Geometry: see drawing. Coordinates: mm, zero at the bounding-box minimum. A direction names the side the tool comes from. Give positions to 0.01 mm unless a question says otherwise; leave off trailing zeros. Loops run counter-clockwise (first coordinate to the right, second up) from the corner with the lowest first, then second, coordinate; pieces in that order, holes last. Notation, with made-up numbers: (89.5, 14.5) -> (94.5, 14.5) arc R33 ccw to (94.5, 44.5) -> close; hole circle Ø5 at (38.5, -7.5). An arc over 180 degrees is marked (long way). Return JSON: item names as keys, results as strings. Group by question number.
(1) Draft query along X for the marked faces 3, 4 and 5. Return one class per face: released by +X, released by -X, zero draft, split by the parting line, or undercut.
(2) Ray query, line 1 (X direction, y = 1.75, z = 10.5); line 2 (X direction, y = 5.75, z = 5.5); line 3 (X direction, y = 3.5, z = 7.75). Return the intervals inside material, ascending. Write a range as from..to.
(3) Cut plane C-C on y = 2.25. Return loops of the section in (x, z), then the cut area to 3 significant figures.
(4) Cut plane B-B on z = 3.5. Return loops of the section in (x, y).
(5) Pin query (flat end, axial travel): pin 1 (2 mm diameter, centred on y = 3, z = 3, fed in from -X); pin 2 (0.5 mm diameter, centred on y = 2, z = 6, fed in from -X); pin 3 (0.9 mm diameter, centred on y = 5, z = 0.5, fed in from -X); pin 4 (3.5 mm diameter, centred on x = 60, y = 2.5, fed in from +Z). Return the tip coordinate at first contact, or that it passes through.
(6) Cut plane D-D on x = 36. Return loops of the section in (y, z).
(7) Cut plane A-A on x = 3.5. Return loops of the section in (y, z).
(8) Access query for the marked faces 1 and 2. Directions: +Z, -Z, +X, -X, +Y, -Y. A direction counts if a zero-diameter tool reaches every point of the face in a straight line with its end or side. Return the directions, or none.
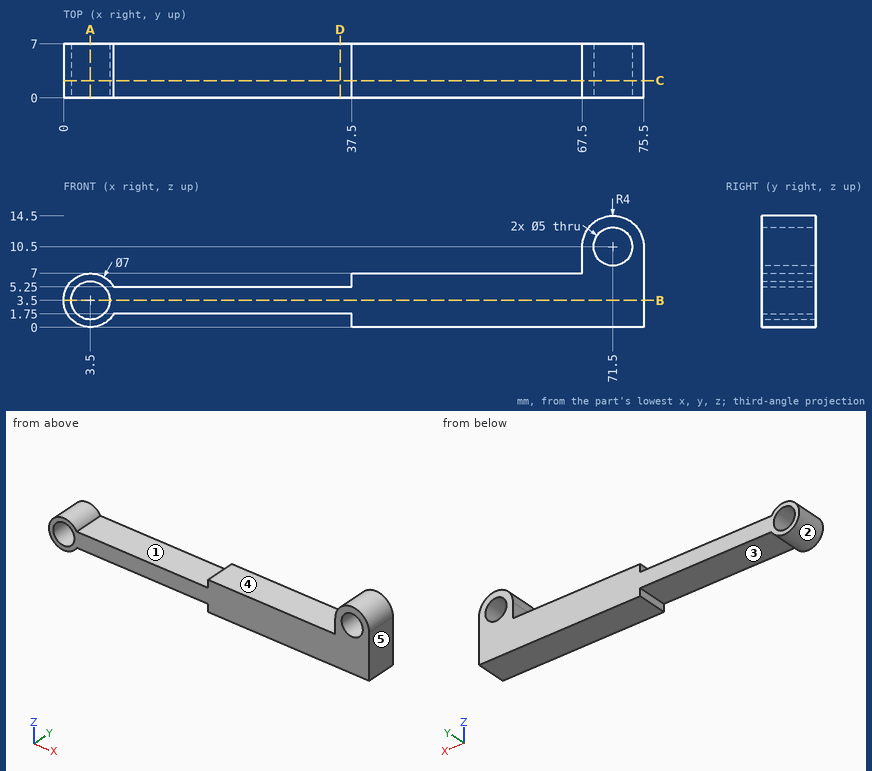
Answers:
{
 "1": {"face 3": "undercut", "face 4": "zero draft", "face 5": "released by +X"},
 "2": {"line 1": "67.5..69, 74..75.5", "line 2": "0.63..2, 5..6.37, 37.5..75.5", "line 3": "67.5..75.5"},
 "3": {"outline": "(6.53, 1.75) -> (37.5, 1.75) -> (37.5, 0) -> (75.5, 0) -> (75.5, 10.5) arc R4 ccw to (67.5, 10.5) -> (67.5, 7) -> (37.5, 7) -> (37.5, 5.25) -> (6.53, 5.25) arc R3.5 ccw (long way) to start; hole circle Ø5 at (3.5, 3.5); hole circle Ø5 at (71.5, 10.5)", "area": "426 mm²"},
 "4": {"outline": "(0, 0) -> (1, 0) -> (1, 7) -> (0, 7) -> close; (6, 0) -> (75.5, 0) -> (75.5, 7) -> (6, 7) -> close"},
 "5": {"pin 1": "x = 0", "pin 2": "x = 0.82", "pin 3": "x = 1.1", "pin 4": "z = 7"},
 "6": {"outline": "(0, 1.75) -> (7, 1.75) -> (7, 5.25) -> (0, 5.25) -> close"},
 "7": {"outline": "(0, 0) -> (7, 0) -> (7, 1) -> (0, 1) -> close; (0, 6) -> (7, 6) -> (7, 7) -> (0, 7) -> close"},
 "8": {"face 1": "+Z, +Y, -Y", "face 2": "+Y, -Y"}
}
